```python
from build123d import *

# Parameters (mm, degrees)
SKETCH1_W               = 12
SKETCH1_H               = 12
SKETCH1_R               = 5.5
BOSS_EXTRUDE1_DEPTH     = 2
BOSS_EXTRUDE1_2_DEPTH   = 2
BOSS_EXTRUDE1_3_DEPTH   = 2
BOSS_EXTRUDE1_4_DEPTH   = 2
BOSS_EXTRUDE1_5_DEPTH   = 2
BOSS_EXTRUDE1_6_DEPTH   = 2
BOSS_EXTRUDE2_START     = -5
BOSS_EXTRUDE2_OUTLINE_R = 1.7
BOSS_EXTRUDE2_DEPTH     = 5
CUT_EXTRUDE1_DEPTH      = 1


# Read off the part's stored shape, not the designer's step: Boss-Extrude2
with BuildPart() as part:
    # Sketch1 → Boss-Extrude1 (new body)
    with BuildSketch(Plane(origin=(0, 0, 0), x_dir=(1, 0, 0), z_dir=(0, 1, 0))):
        with Locations((-2.713611414, -10.664883528)):
            Rectangle(SKETCH1_W, SKETCH1_H)
        with Locations(Location((-2.713611414, -10.664883528, 0), (0, 0, 270))):
            Circle(SKETCH1_R, mode=Mode.SUBTRACT)
    extrude(amount=-BOSS_EXTRUDE1_DEPTH)



with BuildPart() as body_2:
    # Sketch1 → Boss-Extrude1 2 (new body)
    with BuildSketch(Plane(origin=(0, 0, 0), x_dir=(1, 0, 0), z_dir=(0, 1, 0))):
        with Locations((12.886388586, -10.664882884)):
            Rectangle(SKETCH1_W, SKETCH1_H)
        with Locations(Location((12.886388586, -10.664882884, 0), (0, 0, 270))):
            Circle(SKETCH1_R, mode=Mode.SUBTRACT)
    extrude(amount=-BOSS_EXTRUDE1_2_DEPTH)


with BuildPart() as body_3:
    # Sketch1 → Boss-Extrude1 3 (new body)
    with BuildSketch(Plane(origin=(0, 0, 0), x_dir=(1, 0, 0), z_dir=(0, 1, 0))):
        with Locations((5.086388588, -23.66488245)):
            Rectangle(SKETCH1_W, SKETCH1_H)
        with Locations(Location((5.086388588, -23.66488245, 0), (0, 0, 270))):
            Circle(SKETCH1_R, mode=Mode.SUBTRACT)
    extrude(amount=-BOSS_EXTRUDE1_3_DEPTH)


with BuildPart() as body_4:
    # Sketch1 → Boss-Extrude1 4 (new body)
    with BuildSketch(Plane(origin=(0, 0, 0), x_dir=(1, 0, 0), z_dir=(0, 1, 0))):
        with Locations((20.686388588, -23.664882884)):
            Rectangle(SKETCH1_W, SKETCH1_H)
        with Locations(Location((20.686388588, -23.664882884, 0), (0, 0, 270))):
            Circle(SKETCH1_R, mode=Mode.SUBTRACT)
    extrude(amount=-BOSS_EXTRUDE1_4_DEPTH)


with BuildPart() as body_5:
    # Sketch1 → Boss-Extrude1 5 (new body)
    with BuildSketch(Plane(origin=(0, 0, 0), x_dir=(1, 0, 0), z_dir=(0, 1, 0))):
        with Locations((28.486388586, -10.664882884)):
            Rectangle(SKETCH1_W, SKETCH1_H)
        with Locations(Location((28.486388586, -10.664882884, 0), (0, 0, 270))):
            Circle(SKETCH1_R, mode=Mode.SUBTRACT)
    extrude(amount=-BOSS_EXTRUDE1_5_DEPTH)


with BuildPart() as body_6:
    # Sketch1 → Boss-Extrude1 6 (new body)
    with BuildSketch(Plane(origin=(0, 0, 0), x_dir=(1, 0, 0), z_dir=(0, 1, 0))):
        with Locations((36.286388588, -23.664883087)):
            Rectangle(SKETCH1_W, SKETCH1_H)
        with Locations(Location((36.286388588, -23.664883087, 0), (0, 0, 270))):
            Circle(SKETCH1_R, mode=Mode.SUBTRACT)
    extrude(amount=-BOSS_EXTRUDE1_6_DEPTH)


with BuildPart() as part_1:
    add(part.part)

    add(body_2.part)  # Boss-Extrude2 merges body 2

    add(body_3.part)  # Boss-Extrude2 merges body 3

    add(body_4.part)  # Boss-Extrude2 merges body 4

    add(body_5.part)  # Boss-Extrude2 merges body 5

    add(body_6.part)  # Boss-Extrude2 merges body 6
    # Boss-Extrude2 outline → Boss-Extrude2 (add)
    with BuildSketch(Plane(origin=(0, 0, 0), x_dir=(1, 0, 0), z_dir=(0, 1, 0)).offset(BOSS_EXTRUDE2_START)):
        Polygon((42.286388588, -29.664883087), (38.786388588, -29.664883087), (38.786388588, -30.164883087), (54.418988347, -30.16488245), (54.418988347, -4.164883528), (30.986388586, -4.164882884), (30.986388586, -4.664882884), (34.486388586, -4.664882884), (34.486388586, -16.664882884), (22.486388586, -16.664882884), (22.486388586, -4.664882884), (25.986388586, -4.664882884), (25.986388586, -4.164882884), (15.386388586, -4.164882884), (15.386388586, -4.664882884), (18.886388586, -4.664882884), (18.886388586, -16.664882884), (6.886388586, -16.664882884), (6.886388586, -4.664882884), (10.386388586, -4.664882884), (10.386388586, -4.164882884), (-0.213611414, -4.164883528), (-0.213611414, -4.664883528), (3.286388586, -4.664883528), (3.286388586, -16.664883528), (-8.713611414, -16.664883528), (-8.713611414, -4.664883528), (-5.213611414, -4.664883528), (-5.213611414, -4.164883528), (-19.213611414, -4.164883528), (-19.213611414, -30.16488245), (2.586388588, -30.16488245), (2.586388588, -29.66488245), (-0.913611412, -29.66488245), (-0.913611412, -17.66488245), (11.086388588, -17.66488245), (11.086388588, -29.66488245), (7.586388588, -29.66488245), (7.586388588, -30.16488245), (18.186388588, -30.164882884), (18.186388588, -29.664882884), (14.686388588, -29.664882884), (14.686388588, -17.664882884), (26.686388588, -17.664882884), (26.686388588, -29.664882884), (23.186388588, -29.664882884), (23.186388588, -30.164882884), (33.786388588, -30.164882884), (33.786388588, -29.664883087), (30.286388588, -29.664883087), (30.286388588, -17.664883087), (42.286388588, -17.664883087), align=None)
        with Locations((-14.213611414, -17.164882989)):
            Circle(BOSS_EXTRUDE2_OUTLINE_R, mode=Mode.SUBTRACT)
        with Locations((49.418988347, -17.164882989)):
            Circle(BOSS_EXTRUDE2_OUTLINE_R, mode=Mode.SUBTRACT)
    extrude(amount=BOSS_EXTRUDE2_DEPTH)

    # Sketch2 → Cut-Extrude1 (cut)
    with BuildSketch(Plane(origin=(0, -5, 0), x_dir=(-1, 0, 0), z_dir=(0, -1, 0))):
        Polygon((6.798219501, -22.292392997), (8.345014372, -22.292392997), (8.345014372, -22.618034023), (7.083155398, -22.618034023), (7.083155398, -23.5949571), (8.345014372, -23.5949571), (8.345014372, -23.920598125), (7.083155398, -23.920598125), (7.083155398, -25.467392997), (6.798219501, -25.467392997), align=None)
        with BuildLine():
            Line((10.624501552, -22.292392997), (10.624501552, -22.618034023))
            Line((10.624501552, -22.618034023), (9.545179637, -22.618034023))
            Line((9.545179637, -22.618034023), (9.373454877, -23.453125169))
            add(Edge.make_bspline(
                [(9.373454877, -23.453125169), (9.407069849, -23.443844851), (9.47219354, -23.425865702), (9.568314271, -23.405903325), (9.65956577, -23.393869672), (9.718779856, -23.392226555), (9.747433243, -23.391431459)],
                knots=[0, 0, 0, 0, 1.100273476, 2.13160584, 3.095893838, 4, 4, 4, 4], degree=3))
            add(Edge.make_bspline(
                [(9.747433243, -23.391431459), (9.782887778, -23.392198843), (9.852600253, -23.393707713), (9.95459844, -23.408196462), (10.051964708, -23.431001956), (10.144495429, -23.462861287), (10.232361786, -23.50360083), (10.314755359, -23.55449149), (10.392912895, -23.613939584), (10.465432248, -23.682288273), (10.531222156, -23.757510025), (10.589067018, -23.838388951), (10.638200225, -23.924139045), (10.677716053, -24.015579597), (10.709270413, -24.111699686), (10.73027258, -24.213510672), (10.744257737, -24.320052895), (10.745820188, -24.392900612), (10.746616936, -24.430048246)],
                knots=[0, 0, 0, 0, 1.052922333, 2.070308379, 3.05430497, 4.020497103, 4.973039431, 5.925935799, 6.892292201, 7.88610001, 8.88166317, 9.857072816, 10.836096531, 11.812156883, 12.81219415, 13.836441305, 14.89672472, 16, 16, 16, 16], degree=3))
            add(Edge.make_bspline(
                [(10.746616936, -24.430048246), (10.746013618, -24.455921974), (10.744815135, -24.50731977), (10.738720416, -24.583650581), (10.726985874, -24.658365436), (10.711230867, -24.731474249), (10.690781673, -24.802838608), (10.666026603, -24.87266278), (10.635731635, -24.940512173), (10.602501745, -25.007028781), (10.565085297, -25.070708856), (10.523557651, -25.130261865), (10.479683241, -25.186581177), (10.43247427, -25.239062778), (10.381491939, -25.287361801), (10.327353683, -25.331764885), (10.270491502, -25.373022949), (10.210025675, -25.409461241), (10.147303566, -25.442991922), (10.081419397, -25.470499703), (10.013872905, -25.495092824), (9.94369191, -25.514695753), (9.87103538, -25.530055999), (9.795783548, -25.540488687), (9.718331083, -25.548087312), (9.665830179, -25.548562979), (9.639310246, -25.548803254)],
                knots=[0, 0, 0, 0, 1.056347294, 2.098418968, 3.122841568, 4.141288669, 5.149314143, 6.15115421, 7.162517403, 8.180376062, 9.185164535, 10.17417709, 11.141909838, 12.097768115, 13.052685741, 14.0056014, 14.954263652, 15.917497458, 16.885230207, 17.854509472, 18.828990115, 19.81800267, 20.826176721, 21.857883937, 22.917946725, 24, 24, 24, 24], degree=3))
            add(Edge.make_bspline(
                [(9.639310246, -25.548803254), (9.607674382, -25.548176565), (9.545434557, -25.546943629), (9.454248042, -25.534045431), (9.366514079, -25.51557245), (9.282938915, -25.487780977), (9.202773555, -25.452958217), (9.127097232, -25.408947118), (9.053976278, -25.359073217), (8.986383216, -25.300217468), (8.923648742, -25.235886814), (8.867490695, -25.166075239), (8.817476664, -25.09193496), (8.774407565, -25.01310592), (8.737670075, -24.929795253), (8.708809335, -24.841690816), (8.685515399, -24.749252955), (8.675660725, -24.685613699), (8.670655398, -24.653290433)],
                knots=[0, 0, 0, 0, 1.0467383, 2.05933395, 3.04377827, 4.011590433, 4.970194871, 5.932262533, 6.905835911, 7.896367577, 8.894135286, 9.877477877, 10.858688626, 11.851381753, 12.8477658, 13.868841284, 14.917554742, 16, 16, 16, 16], degree=3))
            Line((8.670655398, -24.653290433), (8.955591295, -24.653290433))
            add(Edge.make_bspline(
                [(8.955591295, -24.653290433), (8.962602201, -24.683567644), (8.976077551, -24.741762123), (9.005655623, -24.823524126), (9.041819667, -24.896385136), (9.084822183, -24.961308972), (9.13612114, -25.017922848), (9.19465855, -25.068375469), (9.26028827, -25.113891479), (9.333216414, -25.151830703), (9.410153993, -25.184187358), (9.490678534, -25.205733539), (9.572597477, -25.220883634), (9.628004284, -25.22240016), (9.655846704, -25.223162228)],
                knots=[0, 0, 0, 0, 1.136247022, 2.183929868, 3.172523383, 4.106158343, 5.02341133, 5.958108904, 6.928429099, 7.938127109, 8.96079061, 9.975095812, 10.982467395, 12, 12, 12, 12], degree=3))
            add(Edge.make_bspline(
                [(9.655846704, -25.223162228), (9.683023293, -25.222417665), (9.736534219, -25.220951615), (9.815284548, -25.209667654), (9.891314798, -25.192289), (9.963874758, -25.166281346), (10.034234154, -25.134672208), (10.100613217, -25.094109247), (10.164932256, -25.047427659), (10.225192063, -24.993945573), (10.280382135, -24.935008778), (10.329146616, -24.871982857), (10.369765673, -24.804748289), (10.4039959, -24.734469072), (10.429988536, -24.660374952), (10.448531426, -24.582813172), (10.459419915, -24.501592154), (10.460917771, -24.446193566), (10.461681039, -24.417963911)],
                knots=[0, 0, 0, 0, 1.027316725, 2.022795036, 3.002884548, 3.971462791, 4.93288096, 5.914575861, 6.907176829, 7.935150275, 8.956128384, 9.956726525, 10.942570165, 11.921478529, 12.907843606, 13.90538589, 14.932640048, 16, 16, 16, 16], degree=3))
            add(Edge.make_bspline(
                [(10.461681039, -24.417963911), (10.461083704, -24.392495193), (10.459914506, -24.342643802), (10.450361774, -24.269710237), (10.433745664, -24.20070112), (10.410682573, -24.135283207), (10.381400448, -24.073394799), (10.345617007, -24.014972023), (10.302660711, -23.960784903), (10.25359164, -23.910808086), (10.199836132, -23.864684521), (10.140469308, -23.825365243), (10.076733517, -23.79228726), (10.009396666, -23.76374129), (9.93685708, -23.743239186), (9.860551277, -23.72784689), (9.779655264, -23.718942953), (9.72434614, -23.717707526), (9.695915815, -23.717072484)],
                knots=[0, 0, 0, 0, 1.045622112, 2.046656509, 3.013763289, 3.955457236, 4.890082067, 5.820317437, 6.762574623, 7.722996705, 8.69280354, 9.665887285, 10.63943826, 11.638615906, 12.663482002, 13.728887084, 14.832589034, 16, 16, 16, 16], degree=3))
            add(Edge.make_bspline(
                [(9.695915815, -23.717072484), (9.671306001, -23.717599164), (9.620492978, -23.718686622), (9.5425487, -23.726693516), (9.460641208, -23.73961059), (9.375084487, -23.757378115), (9.285621598, -23.780629163), (9.192441334, -23.808491603), (9.095347778, -23.841803701), (9.0299267, -23.866960781), (8.996296424, -23.879892997)],
                knots=[0, 0, 0, 0, 0.817624296, 1.688186739, 2.600797293, 3.572016777, 4.590301741, 5.671205678, 6.80286297, 8, 8, 8, 8], degree=3))
            Line((8.996296424, -23.879892997), (9.321937449, -22.292392997))
            Line((9.321937449, -22.292392997), (10.624501552, -22.292392997))
        make_face()
    extrude(amount=-CUT_EXTRUDE1_DEPTH, mode=Mode.SUBTRACT)


solid = part_1.part
```
For this review, take the finished solid that the model builds, in its own axes (mm). A direction names the side the tool comes from. Give positions to 0.01 mm unless a question says otherwise; leave off trailing zeros. Order: outer loops, then holes, each group sorted by start corner. A loop starts at its lowest first (then second) coordinate and runs counter-clockwise, first axis right, second up.
1) Take a section at C-C (y = -1.05). State how many separate pieces and enclosed holes the cut face has, then the cut area to 3 significant figures.
2) Insertion check: pin 1 (0.6 mm diameter, centred on x = -3, y = -1, fed in from -Z); pin 2 (1 mm diameter, centred on x = 5.5, y = -4, fed in from +Z); pin 3 (8 mm diameter, centred on x = 11, z = 11.5, fed in from -Y). Each pin has a flat end and moves straight along its axis. Give the tip position at first contact, or say it passes through.
3) For faces 1 (the face through (-3, -1, 4.665)), 2 (the face through (14.686, -4, 24)), 3 (the face through (5, -3, 4.165)), list the 3-axis set-ups (+Z, -Z, +X, -X, +Y, -Y) from which the entire face can be reached by the end or side of a thin tool; tool diameter is ignored.
4) Take a section at A-A (z = 26.25). Give the boundary of the cut face in (x, y).
5) The part is to be moulded in two halves that separate along X. For faces 4 (the face through (21, -3, 4.165)), 5 (the face through (36, -4, 17.665)), 6 (the face through (-0.914, -4, 24)), say which applies: released by +X, released by -X, zero draft, split by the parting line, or undercut.
6) Take a section at B-B (z = 13). Give the boundary of the cut face in (x, y).
7) Wall thickness on line 1 (X direction, y = -3.7, z = 25); line 2 (X direction, y = -3.9, z = 13.5); line 3 (Z direction, x = 17.5, y = -2.95): over which ranges is each line inside the solid? List them lowest first.
Derived:
1. separate pieces: 1
1. enclosed holes: 8
1. area: 1,310 mm2
2. pin 1: stops at z = 4.66
2. pin 2: stops at z = 17.66
2. pin 3: stops at y = -2
3. face 1: -Z, +Y, -Y
3. face 2: -Y
3. face 3: -Z, +X, -X, +Y, -Y
4. outline: (-19.21, -5) - (-0.91, -5) - (-0.91, -2) - (0.23, -2) - (0.23, 0) - (-19.21, 0) - close; (9.94, -2) - (11.09, -2) - (11.09, -5) - (14.69, -5) - (14.69, -2) - (15.83, -2) - (15.83, 0) - (9.94, 0) - close; (25.54, -2) - (26.69, -2) - (26.69, -5) - (30.29, -5) - (30.29, -2) - (31.43, -2) - (31.43, 0) - (25.54, 0) - close; (41.14, -2) - (42.29, -2) - (42.29, -5) - (54.42, -5) - (54.42, 0) - (41.14, 0) - close
5. face 4: zero draft
5. face 5: undercut
5. face 6: undercut
6. outline: (-19.21, -5) - (-8.71, -5) - (-8.71, -2) - (-7.69, -2) - (-7.69, 0) - (-19.21, 0) - close; (2.27, -2) - (3.29, -2) - (3.29, -5) - (6.89, -5) - (6.89, -2) - (7.91, -2) - (7.91, 0) - (2.27, 0) - close; (17.87, -2) - (18.89, -2) - (18.89, -5) - (22.49, -5) - (22.49, -2) - (23.51, -2) - (23.51, 0) - (17.87, 0) - close; (33.47, -2) - (34.49, -2) - (34.49, -5) - (54.42, -5) - (54.42, 0) - (33.47, 0) - close
7. line 1: x = -19.21 to -0.91, 11.09 to 14.69, 26.69 to 30.29, 42.29 to 54.42
7. line 2: x = -19.21 to -8.71, 3.29 to 6.89, 18.89 to 22.49, 34.49 to 54.42
7. line 3: z = 4.16 to 4.66, 16.66 to 17.66, 29.66 to 30.16
